Verification items for this drawing (mm, ordinates from the low corner). A direction names the side the tool comes from. Give positions to 0.01 mm unless a question says otherwise; leave off trailing zeros. Order: outer loops, then holes, each group sorted by start corner. A loop starts at its lowest first (then second) coordinate and runs counter-clockwise, first axis right, second up.
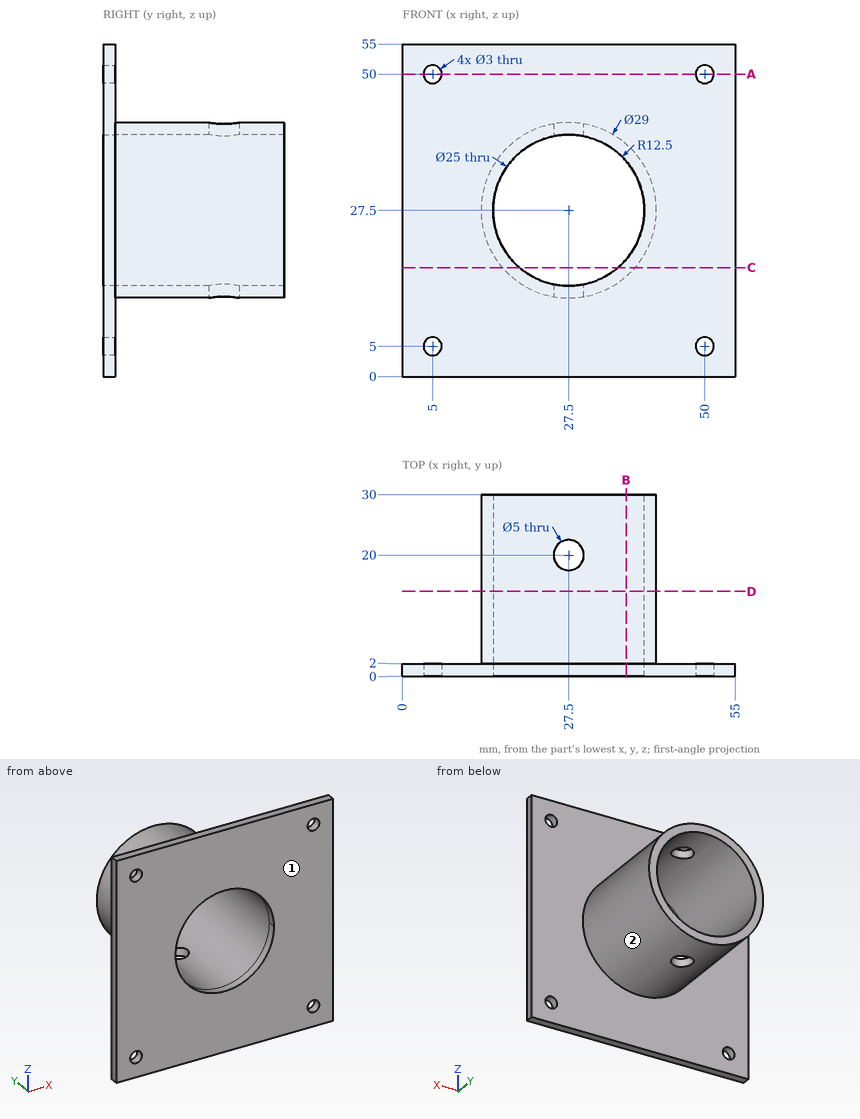
Q1. Cross-section at B-B, the plane x = 37. Record the boundary of the cut face in (y, z).
Q2. Thickness scan on L1, parallel to X at y = 1.1, z = 50; L2, parallel to X at y = 1, z = 27. Record the ranges inside material, lowest first.
Q3. Cross-section at D-D, the plane y = 14. Record the boundary of the cut face in (x, z).
Q4. Gauge pin test, flat ends, axial feed: P1, Ø6, axis at y = 7.5, z = 22, coming from the +X side; P2, Ø1.5, axis at x = 20, y = 6, coming from the -Z side; P3, Ø5, axis at y = 23, z = 19, coming from the +X side; P4, Ø3.5, axis at x = 5, z = 5, coming from the -Y side. Record the tip position at first contact, or that the pin passes through.
Q5. Cross-section at C-C, the plane z = 18. Record the boundary of the cut face in (x, y), and give its area (3 significant figures).
Q6. Access from +Z, -Z, +X, -X, +Y, -Y to the whole of each face (thin tool, end or side, straight path). Record for the marked faces 1 and 2.
Q7. Cross-section at A-A, the plane z = 50. Record the boundary of the cut face in (x, y).
Answers follow:
1. outline: (0, 0) - (2, 0) - (2, 16.55) - (30, 16.55) - (30, 19.38) - (0, 19.38) - close; (0, 35.62) - (30, 35.62) - (30, 38.45) - (2, 38.45) - (2, 55) - (0, 55) - close
2. L1: x = 0 to 3.5, 6.5 to 48.5, 51.5 to 55
2. L2: x = 0 to 15.01, 39.99 to 55
3. outline: circle Ø29 at (27.5, 27.5); hole circle Ø25 at (27.5, 27.5)
4. P1: stops at x = 41.78
4. P2: stops at z = 14.67
4. P3: stops at x = 40.7
4. P4: stops at y = 0
5. outline: (0, 0) - (19.38, 0) - (19.38, 30) - (16.55, 30) - (16.55, 2) - (0, 2) - close; (35.62, 0) - (55, 0) - (55, 2) - (38.45, 2) - (38.45, 30) - (35.62, 30) - close
5. area: 236 mm2
6. face 1: +Z, -Z, +X, -X, -Y
6. face 2: +Y
7. outline: (0, 0) - (3.5, 0) - (3.5, 2) - (0, 2) - close; (6.5, 0) - (48.5, 0) - (48.5, 2) - (6.5, 2) - close; (51.5, 0) - (55, 0) - (55, 2) - (51.5, 2) - close
